For this review, use the dimensioned drawing (mm, ordinates from the lowest corner) and the shaded views. A direction names the side the tool comes from. Give positions to 0.01 mm unless a question says otherwise; leave off trailing zeros. Write each loop counter-clockwise with the first axis right and the second up, starting at its lowest first coordinate (ties: lowest second). Pieces come first, ordered by that corner, then holes. Notation, with made-up numbers: M 26.25,54.25 L 72.25,54.25 A19 cw 72.25,91.25 Z; hole C 51,16 d1. An arc over 180 degrees is marked long. Use a Markdown table: item, result. Add a question column.
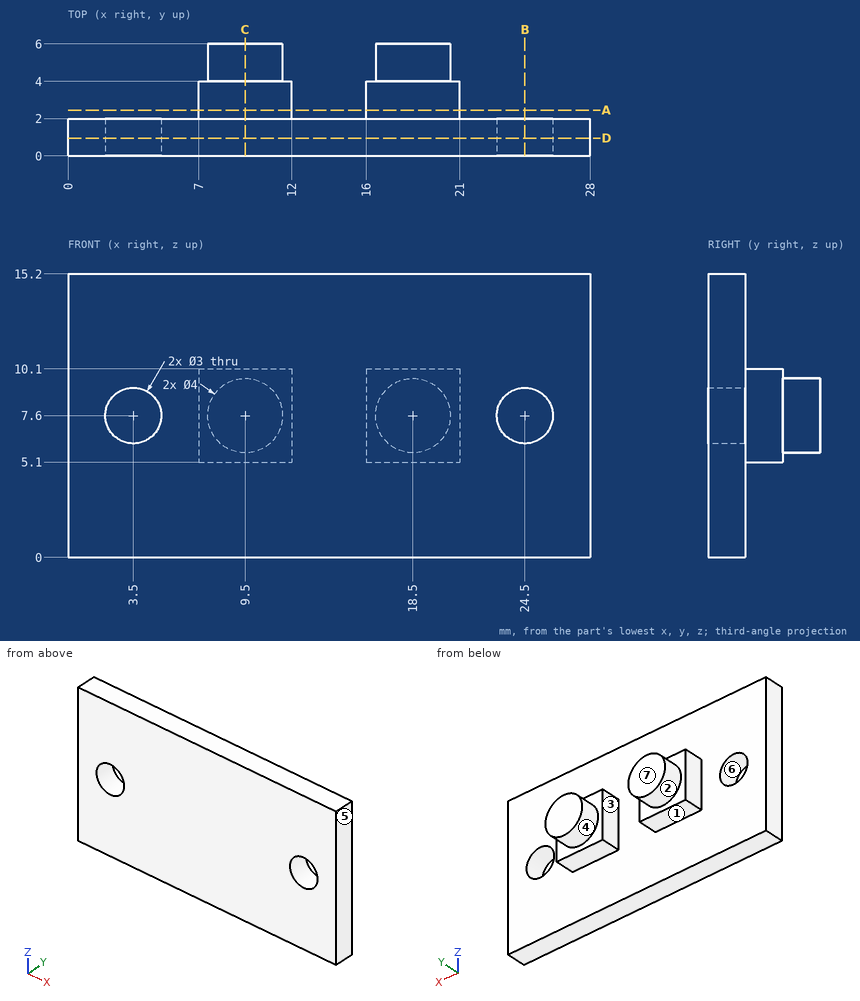
(1) Add section D-D on y = 0.95. Give the boundary of the cut face in (x, z).
(2) Add section B-B on x = 24.5. Give the boundary of the cut face in (y, z), then the cut area to 3 significant figures.
(3) The part is to be moulded in two halves that separate along X. For the marked faces 4, 5, 6 and 7, say which applies: released by +X, released by -X, zero draft, split by the parting line, or undercut.
(4) Wall thickness on L1, parallel to X at y = 0.9, z = 7.6; L2, parallel to Y at x = 5.75, z = 11.75; L3, parallel to X at y = 5.15, z = 7.25: over which ranges is each line inside the solid? List them lowest first.
(5) Add section A-A on y = 2.45. Give the boundary of the cut face in (x, z), then the cut area to 3 significant figures.
(6) For pin 1 (0.6 mm diameter, centred on x = 18.5, y = 3.5, fed in from +Z); pin 2 (0.6 mm diameter, centred on y = 3.5, z = 7, fed in from -X); pin 3 (1.6 mm diameter, centred on y = 3.5, z = 9, fed in from +X); pin 4 (1 mm diameter, centred on x = 13.5, y = 5, fed in from +Z), all flat-tipped, find the tip position at first contact; note any pin that passes through.
(7) Machinability: for the marked faces 1, 2 and 3, which of the approach directions +Z, -Z, +X, -X, +Y, -Y give a long, thin tool a straight path to every point of the face, cutting with its end or side? Answer none if there is none.
(8) Add section C-C on x = 9.5. Give the boundary of the cut face in (y, z), then the cut area to 3 significant figures.
From the geometry:
| question | item | result |
|---|---|---|
| 1 | outline | M 0,0 L 28,0 L 28,15.2 L 0,15.2 Z; hole C 3.5,7.6 d3; hole C 24.5,7.6 d3 |
| 2 | outline | M 0,0 L 2,0 L 2,6.1 L 0,6.1 Z; M 0,9.1 L 2,9.1 L 2,15.2 L 0,15.2 Z |
| 2 | area | 24.4 mm^2 |
| 3 | face 4 | undercut |
| 3 | face 5 | released by +X |
| 3 | face 6 | undercut |
| 3 | face 7 | zero draft |
| 4 | L1 | x = 0 to 2, 5 to 23, 26 to 28 |
| 4 | L2 | y = 0 to 2 |
| 4 | L3 | x = 7.53 to 11.47, 16.53 to 20.47 |
| 5 | outline | M 7,5.1 L 12,5.1 L 12,10.1 L 7,10.1 Z; M 16,5.1 L 21,5.1 L 21,10.1 L 16,10.1 Z |
| 5 | area | 50.0 mm^2 |
| 6 | pin 1 | stops at z = 10.1 |
| 6 | pin 2 | stops at x = 7 |
| 6 | pin 3 | stops at x = 21 |
| 6 | pin 4 | passes through |
| 7 | face 1 | -Z, +X, -X, +Y |
| 7 | face 2 | +Y |
| 7 | face 3 | +Z, -Z, +Y |
| 8 | outline | M 0,0 L 2,0 L 2,5.1 L 4,5.1 L 4,5.6 L 6,5.6 L 6,9.6 L 4,9.6 L 4,10.1 L 2,10.1 L 2,15.2 L 0,15.2 Z |
| 8 | area | 48.4 mm^2 |
